Build history of the part. All positions in model axes, mm. Face numbers are marked on the shaded views. A direction names the side the tool comes from. Give positions to 0.01 mm unless a question says otherwise; leave off trailing zeros. Write each loop counter-clockwise with the first axis right and the second up, starting at its lowest first coordinate (ties: lowest second). Pieces come first, ordered by that corner, then holes. Notation, with made-up numbers: (7.5, 62) -> (42.5, 62) arc R23 cw to (42.5, 77) -> close; hole circle Ø6 at (-33.75, 37.5). An arc over 180 degrees is marked (long way). Write item = value, one per line. Start each with the question number.
Q1. Drop flat-ended pins along their axis: P1, Ø10.5, axis at y = 56.5, z = 111, coming from the -X side; P2, Ø2, axis at x = 144, y = 43, coming from the +Z side; P3, Ø9.5, axis at x = 16.5, y = 57.5, coming from the +Z side; P4, Ø12, axis at x = 146.5, z = 63, coming from the +Y side. Give the stop position or say it passes through.
Q2. Saw through at B-B, the plane y = 71.5. List the corners of the cut face in (x, z).
Q3. Saw through at C-C, the plane z = 98. List the corners of the cut face in (x, y), then the cut area to 3 significant figures.
Q4. Mould opens along Z. For the marked faces 4, 5 and 6 say: pulls with the +Z half, pulls with the -Z half, needs draft (parallel to the pull), parting line crosses it, or undercut.
Q5. Wall check: line 1 (X direction, y = 9, z = 66); line 2 (X direction, y = 53, z = 39.5); line 3 (X direction, y = 39, z = 113). Give the ranges that are in metal, low to high.
Q6. Tool access for the marked faces 1, 2 and 3: list every direction of +Z, -Z, +X, -X, +Y, -Y with a clear straight run to the whole face (end or side of a thin tool).
Autodesk Inventor part; units mm, degrees
ref_plane "YZ Plane" through (0, 0, 0) normal (1, 0, 0) x (0, 1, 0)
ref_plane "XZ Plane" through (0, 0, 0) normal (0, 1, 0) x (-1, 0, 0)
ref_plane "XY Plane" through (0, 0, 0) normal (0, 0, 1) x (1, 0, 0)
sketch "Esboço3" plane through (0, 0, 0) normal (0, 0, 1) x (1, 0, 0)
  line L0 (0, 0) -> (204.6, 0)
  line L1 (204.6, 0) -> (204.6, 80)
  line L2 (204.6, 80) -> (0, 80)
  line L3 (0, 80) -> (0, 0)
  dimension "d4" = 204.6
  dimension "d5" = 80
extrude "Extrusão2" add sketch "Esboço3" along normal blind 200
sketch "Esboço7" plane through (0, 80, 0) normal (0, 1, 0) x (1, 0, 0)
  line L0 (0, 0) -> (5, 0)
  line L1 (0, 0) -> (204.6, 0)
  line L2 (5, -5) -> (5, -80)
  line L3 (5, -80) -> (35, -80)
  line L4 (5, -5) -> (35, -5)
  line L5 (35, -5) -> (35, -80)
  line L6 (35, -80) -> (5, -80)
  line L7 (5, -80) -> (5, -5)
  line L8 (204.6, 0) -> (204.6, -200)
  line L9 (199.6, -5) -> (199.6, -80)
  line L10 (199.6, -80) -> (169.6, -80)
  line L11 (199.6, -5) -> (169.6, -5)
  line L12 (169.6, -5) -> (169.6, -80)
  line L13 (169.6, -80) -> (199.6, -80)
  line L14 (199.6, -80) -> (199.6, -5)
extrude "Extrusão3" cut sketch "Esboço7" against normal through all
sketch "Esboço8" plane through (0, 80, 0) normal (0, 1, 0) x (1, 0, 0)
  line L0 (35, -5) -> (35, -80)
  line L1 (35, -80) -> (36.6, -80)
  line L2 (169.6, -80) -> (168, -80)
  line L3 (45.7132, 0) -> (45.7132, -5)
  line L4 (0, 0) -> (204.6, 0)
  line L5 (36.6, -80) -> (168, -80)
  line L6 (168, -80) -> (168, -5)
  line L7 (168, -5) -> (36.6, -5)
  line L8 (36.6, -5) -> (36.6, -80)
  dimension "d29" = 1.6
  dimension "d30" = 1.6
extrude "Extrusão4" cut sketch "Esboço8" against normal blind 66.25
sketch "Esboço9" plane through (0, 80, 0) normal (0, 1, 0) x (1, 0, 0)
  line L0 (35, -80) -> (5, -80)
  line L1 (168, -80) -> (36.6, -80)
  line L2 (36.6, -80) -> (36.6, -85)
  line L3 (168, -80) -> (168, -85)
  line L4 (199.6, -80) -> (169.6, -80)
  line L5 (5, -120) -> (5, -85)
  line L6 (36.6, -85) -> (5, -85)
  line L7 (5, -120) -> (140.4393, -120)
  line L8 (199.6, -85) -> (168, -85)
  line L9 (36.6, -80) -> (168, -80)
  line L10 (140.4393, -120) -> (199.6, -120)
  line L11 (199.6, -120) -> (199.6, -85)
extrude "Extrusão5" cut sketch "Esboço9" against normal blind 66.25
chamfer "Chanfro1" distance 80 angle 45 1 edges at (102.3, 80, 200)
properties part number "chassi1"
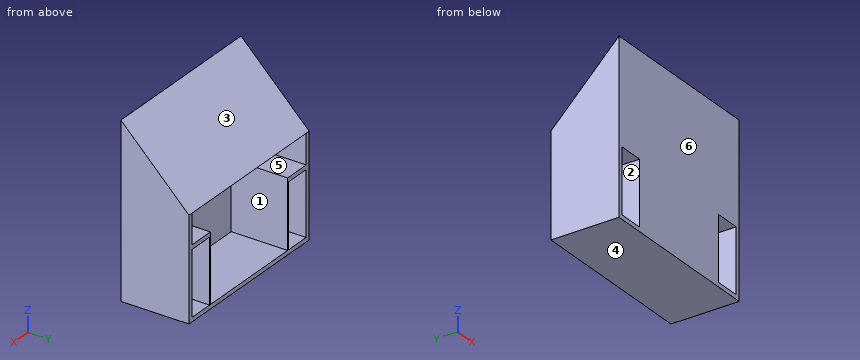
Report:
q1.P1 = 0
q1.P2 = 158
q1.P3 = 147.25
q1.P4 = 13.75
q2.outline = (0, 0) -> (204.6, 0) -> (204.6, 128.5) -> (0, 128.5) -> close; hole (5, 5) -> (35, 5) -> (35, 80) -> (5, 80) -> close; hole (5, 85) -> (36.6, 85) -> (36.6, 5) -> (168, 5) -> (168, 85) -> (199.6, 85) -> (199.6, 120) -> (5, 120) -> close; hole (169.6, 5) -> (199.6, 5) -> (199.6, 80) -> (169.6, 80) -> close
q3.outline = (0, 0) -> (204.6, 0) -> (204.6, 80) -> (199.6, 80) -> (199.6, 13.75) -> (5, 13.75) -> (5, 80) -> (0, 80) -> close
q3.area = 3,480 mm2
q4.face_4 = pulls with the -Z half
q4.face_5 = undercut
q4.face_6 = needs draft
q5.line_1 = 0 to 5, 35 to 169.6, 199.6 to 204.6
q5.line_2 = 0 to 5, 35 to 36.6, 168 to 169.6, 199.6 to 204.6
q5.line_3 = 0 to 5, 199.6 to 204.6
q6.face_1 = +Y
q6.face_2 = +Y, -Y
q6.face_3 = +Z, +X, -X, +Y
